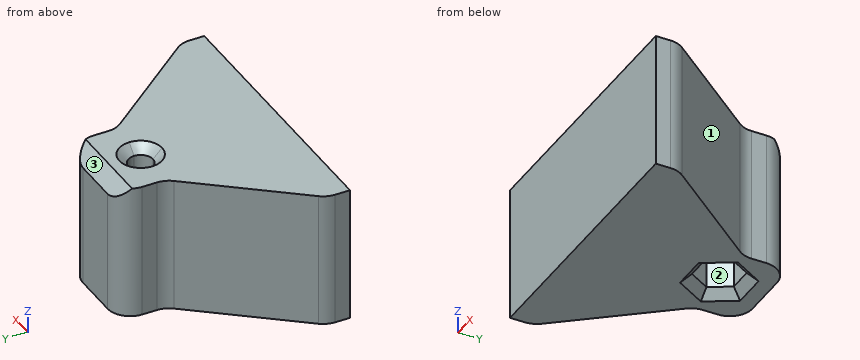
from build123d import *

# Parameters (mm, degrees)
BOSS_EXTRUDE1_DEPTH = 38.1
CUT_EXTRUDE1_DEPTH  = 19.05
CHAMFER1_SIZE       = 2.54
CHAMFER2_SIZE       = 2.54
FILLET1_R           = 6.35
CHAMFER3_SIZE       = 3.81


with BuildPart() as part:
    # Sketch1 → Boss-Extrude1 (new body)
    with BuildSketch(Plane.XY):
        with BuildLine():
            Line((0, 3.429), (0, 12.7))
            Line((0, 12.7), (-12.7, 12.7))
            Line((-12.7, 12.7), (-12.7, 0))
            Line((-12.7, 0), (-38.1, -31.75))
            Line((-38.1, -31.75), (-38.1, -38.1))
            Line((-38.1, -38.1), (0, -38.1))
            Line((0, -38.1), (0, -3.429))
            ThreePointArc((0, -3.429), (-3.429, 0), (0, 3.429))
        make_face()
        with BuildLine():
            Line((12.7, 12.7), (0, 12.7))
            Line((0, 12.7), (0, 3.429))
            ThreePointArc((0, 3.429), (2.424669153, 2.424669153), (3.429, 0))
            ThreePointArc((3.429, 0), (2.424669153, -2.424669153), (0, -3.429))
            Line((0, -3.429), (0, -38.1))
            Line((0, -38.1), (38.1, -38.1))
            Line((38.1, -38.1), (38.1, -31.75))
            Line((38.1, -31.75), (12.7, 0))
            Line((12.7, 0), (12.7, 12.7))
        make_face()
    extrude(amount=BOSS_EXTRUDE1_DEPTH)

    # Sketch2 → Cut-Extrude1 (cut)
    with BuildSketch(Plane(origin=(0, 0, 0), x_dir=(-1, 0, 0), z_dir=(0, 0, -1))):
        Polygon((6.745760545, 0), (3.372880273, 5.842), (-3.372880273, 5.842), (-6.745760545, 0), (-3.372880273, -5.842), (3.372880273, -5.842), align=None)
    extrude(amount=-CUT_EXTRUDE1_DEPTH, mode=Mode.SUBTRACT)

    # Chamfer1
    chamfer1_edges = [part.edges().sort_by_distance(p)[0] for p in [
        (-5.059320409, -2.921, 0),
        (-5.059320409, 2.921, 0),
        (0, 5.842, 0),
        (5.059320409, 2.921, 0),
        (5.059320409, -2.921, 0),
        (0, -5.842, 0),
    ]]
    chamfer(chamfer1_edges, length=CHAMFER1_SIZE)

    # Chamfer2
    chamfer2_edges = [part.edges().sort_by_distance(p)[0] for p in [
        (0, 3.429, 38.1),
    ]]
    chamfer(chamfer2_edges, length=CHAMFER2_SIZE)

    # Fillet1
    fillet1_edges = [part.edges().sort_by_distance(p)[0] for p in [
        (12.7, 0, 19.05),
        (38.1, -31.75, 19.05),
        (-38.1, -31.75, 19.05),
        (-12.7, 0, 19.05),
        (-12.7, 12.7, 19.05),
        (12.7, 12.7, 19.05),
    ]]
    fillet(fillet1_edges, radius=FILLET1_R)

    # Chamfer3
    # the kernel refuses this chamfer: 3.81 mm, written as the material it takes off along each edge
    with BuildSketch(Plane(origin=(-16.148112184, 12.7, 38.1), x_dir=(0, -0.9996219169112968, 0.027495876610586386), z_dir=(1, 0, 0))) as chamfer3_piece_1:
        Polygon((CHAMFER3_SIZE * 0.999621916911, CHAMFER3_SIZE * 0.0274958766106), (-CHAMFER3_SIZE * 0.0274958766106, CHAMFER3_SIZE * 0.999621916911), (0, 0), align=None)
    extrude(amount=32.296224368, mode=Mode.SUBTRACT)


solid = part.part
CAD build for the part. Positions are in the model's coordinates, mm. Face numbers are marked on the shaded views. Round coordinates to 2 decimals unless told otherwise and drop trailing zeros. Write each loop counter-clockwise with the first axis right and the second up, starting at its lowest first coordinate (ties: lowest second). Pieces come first, ordered by that corner, then holes. Notation, with made-up numbers: M 58,6.5 L 69,6.5 A24 cw 69,21.5 Z; hole C 49,74.5 d7. An arc over 180 degrees is marked long. Put each result on its own line as item: value. Start each with the question number.
1) Saw through at C-C, the plane x = 31.5. Write the cut outline in (y, z).
2) Saw through at D-D, the plane z = 28. Write the cut outline in (x, y), and give its area (3 significant figures).
3) Pin check, flat tips, straight feed: pin 1 Ø3 at (y, z) = (-29.5, 7) entering from -X; pin 2 Ø4 at (y, z) = (-3.5, 14.5) entering from -X; pin 3 Ø1.2 at (y, z) = (5, 9.5) entering from -X. Stop position of each tip, or through.
4) Pull direction X, two halves, no side cores. Call the marked faces 1, 2 and 3: pulls with the +X half, pulls with the -X half, needs draft (parallel to the pull), parting line crosses it, or undercut.
5) Saw through at A-A, the plane z = 7. Write the cut outline in (x, y).
6) Saw through at B-B, the plane y = -9.5. Write the cut outline in (x, z), and give its area (3 significant figures).
7) Drill centre lines: probe 1 along Y at (x, z) = (-2, 16); probe 2 along Y at (x, z) = (-3, 26.5); probe 3 along X at (y, z) = (-2.5, 19.5). Where is each one in solid material? Low to high. Write a range as [from, to].
Resolved:
1. outline: M -38.1,0 L -23.5,0 L -23.5,38.1 L -38.1,38.1 Z
2. outline: M -38.1,-38.1 L 38.1,-38.1 L 38.1,-33.98 A6.35 ccw 36.71,-30.01 L 14.09,-1.74 A6.35 cw 12.7,2.23 L 12.7,6.35 A6.35 ccw 6.35,12.7 L -6.35,12.7 A6.35 ccw -12.7,6.35 L -12.7,2.23 A6.35 cw -14.09,-1.74 L -36.71,-30.01 A6.35 ccw -38.1,-33.98 Z; hole C 0,0 d6.86
2. area: 2,370 mm²
3. pin 1: x = -37.36
3. pin 2: x = -17.1
3. pin 3: x = -12.7
4. face 1: pulls with the +X half
4. face 2: undercut
4. face 3: needs draft
5. outline: M -38.1,-38.1 L 38.1,-38.1 L 38.1,-33.98 A6.35 ccw 36.71,-30.01 L 14.09,-1.74 A6.35 cw 12.7,2.23 L 12.7,6.35 A6.35 ccw 6.35,12.7 L -6.35,12.7 A6.35 ccw -12.7,6.35 L -12.7,2.23 A6.35 cw -14.09,-1.74 L -36.71,-30.01 A6.35 ccw -38.1,-33.98 Z; hole M -6.75,0 L -3.37,-5.84 L 3.37,-5.84 L 6.75,0 L 3.37,5.84 L -3.37,5.84 Z
6. outline: M -20.3,0 L 20.3,0 L 20.3,38.1 L -20.3,38.1 Z
6. area: 1,550 mm²
7. probe 1: [-38.1, -5.84], [5.84, 12.7]
7. probe 2: [-38.1, -1.66], [1.66, 12.7]
7. probe 3: [-14.7, -2.35], [2.35, 14.7]
